from build123d import *

# Parameters (mm, degrees)
F0_W     = 76.2
F0_H     = 76.2
F2_DEPTH = 6.35
F3_DEPTH = 6.35
F4_R     = 2.54
F6_DEPTH = 3.175
F8_DEPTH = 2.778125


with BuildPart() as f2:
    # F0 (on Top) → F2 (new body)
    with BuildSketch(Plane.XY):
        Rectangle(F0_W, F0_H)
    extrude(amount=-F2_DEPTH)

    # F1 (on Front) → F3 (join, symmetric)
    with BuildSketch(Plane.XZ):
        with BuildLine():
            Line((18.72926, 44.45), (25.395371, 51.253571))
            ThreePointArc((25.395371, 51.253571), (-28.575, 28.575), (25.395371, 5.896429))
            Line((25.395371, 5.896429), (18.72926, 12.7))
            ThreePointArc((18.72926, 12.7), (-19.05, 28.575), (18.72926, 44.45))
        make_face()
    extrude(amount=F3_DEPTH, both=True)

    # F4
    f4_edges = [f2.edges().sort_by_distance(p)[0] for p in [
        (25.395371, 0, 51.253571),
        (18.72926, 0, 44.45),
        (18.72926, 0, 12.7),
        (25.395371, 0, 5.896429),
        (3.175, -6.35, 0),
        (3.175, 6.35, 0),
    ]]
    fillet(f4_edges, radius=F4_R)

    # F5 (on face) → F6 (cut)
    with BuildSketch(Plane(origin=(0, 0, -6.35), x_dir=(1, 0, 0), z_dir=(0, 0, -1))):
        Polygon((38.1, 14.2875), (38.1, 23.8125), (31.75, 27.478674), (31.75, 10.621326), align=None)
        Polygon((31.75, -10.621326), (31.75, -27.478674), (38.1, -23.8125), (38.1, -14.2875), align=None)
    extrude(amount=-F6_DEPTH, mode=Mode.SUBTRACT)

    # F7 (on face) → F8 (join)
    with BuildSketch(Plane(origin=(0, 0, -6.35), x_dir=(1, 0, 0), z_dir=(0, 0, -1))):
        Polygon((-38.1, 14.485938), (-38.1, 23.614063), (-44.45, 27.280237), (-44.45, 10.819763), align=None)
        Polygon((-38.1, -23.614063), (-38.1, -14.485938), (-44.45, -10.819763), (-44.45, -27.280237), align=None)
    extrude(amount=-F8_DEPTH)


solid = f2.part
Model file for the job. Use its own axes, mm. A direction names the side the tool comes from. Coordinates: 2 decimals unless noted, no trailing zeros. Loops run counter-clockwise (first coordinate to the right, second up) from the corner with the lowest first, then second, coordinate; pieces in that order, holes last. Notation, with made-up numbers: (78.25, -21.5) -> (135.25, -21.5) arc R19 ccw to (135.25, 11.5) -> close; hole circle Ø9 at (51.25, 24). An arc over 180 degrees is marked (long way). Use one line per item in the form item = value. Start each with the question number.
(1) Cut at D-D on x = 4. Give the cut face in (y, z), and give its area (3 significant figures).
(2) Cut at C-C on x = 27. Give the cut face in (y, z), and give its area (3 significant figures).
(3) Cut at B-B on y = 21.5. Give the cut face in (x, z) (3 decimals).
(4) Flat gauge pins, fed straight in: pin 1 (5 mm diameter, centred on x = -42.5, y = 22, fed in from +Z); pin 2 (1.9 mm diameter, centred on x = 35.5, y = -16, fed in from -Z) (3 decimals); pin 3 (1.6 mm diameter, centred on y = 20, z = -5, fed in from +X). Where does each tip first touch, or does it go through?
(5) Probe probe 1 along Z at (x, y) = (19.5, 0); probe 2 along Z at (x, y) = (24, -0.5); probe 3 along X at (y, z) = (-33, -1). List the from-to ranges inside material, lowest first. Write a range as from..to.
(6) Pull direction X, two halves, no side cores. Call faces 5 (the flat face through (35, -25.6, -4.8)), 6 (the flat face through (38.1, -1, -3)), 7 (the flat face through (-1, 17, 0)): pulls with the +X half, pulls with the -X half, needs draft (parallel to the pull), parting line crosses it, or undercut.
(7) Tool access for faces 1 (the flat face through (-41.319, -12.627, -4.98)), 2 (the flat face through (31.75, -19, -5)), 3 (the flat face through (-14, -6.35, 45)), 4 (the flat face through (-14, 6.35, 45)): list every direction of +Z, -Z, +X, -X, +Y, -Y with a clear straight run to the whole face (end or side of a thin tool).
(8) Cut at A-A on x = -26. Give the cut face in (y, z), and give its area (3 significant figures).
Values:
q1.outline = (-38.1, -6.35) -> (38.1, -6.35) -> (38.1, 0) -> (8.89, 0) arc R2.54 cw to (6.35, 2.54) -> (6.35, 6.37) -> (-6.35, 6.37) -> (-6.35, 2.54) arc R2.54 cw to (-8.89, 0) -> (-38.1, 0) -> close; (-6.35, 50.78) -> (6.35, 50.78) -> (6.35, 60.31) -> (-6.35, 60.31) -> close
q1.area = 689 mm2
q2.outline = (-38.1, -6.35) -> (38.1, -6.35) -> (38.1, 0) -> (-38.1, 0) -> close
q2.area = 484 mm2
q3.outline = (-44.45, -6.35) -> (31.75, -6.35) -> (31.75, -3.175) -> (38.1, -3.175) -> (38.1, 0) -> (-38.1, 0) -> (-38.1, -3.572) -> (-44.45, -3.572) -> close
q4.pin_1 = -3.57
q4.pin_2 = -3.175
q4.pin_3 = 31.75
q5.probe_1 = -6.35..0, 1.34..11.58, 45.57..55.81
q5.probe_2 = -6.35..0, 4.88..7.14, 50.01..52.27
q5.probe_3 = -38.1..38.1
q6.face_5 = undercut
q6.face_6 = pulls with the +X half
q6.face_7 = needs draft
q7.face_1 = +Z, -Z
q7.face_2 = -Z
q7.face_3 = +Z, +X, -X, -Y
q7.face_4 = +Z, +X, -X, +Y
q8.outline = (-38.1, -6.35) -> (38.1, -6.35) -> (38.1, 0) -> (-38.1, 0) -> close; (-6.35, 16.05) -> (6.35, 16.05) -> (6.35, 41.1) -> (-6.35, 41.1) -> close
q8.area = 802 mm2
